from build123d import *

# Parameters (mm, degrees)
SKETCH1_W           = 60.96
SKETCH1_H           = 60.96
SKETCH1_R           = 1
SKETCH1_R_2         = 0.5
BOSS_EXTRUDE1_DEPTH = 1.5
SKETCH1_3_R         = 0.5
CUT_EXTRUDE1_DEPTH  = 0.75


with BuildPart() as part:
    # Sketch1 → Boss-Extrude1 (new body)
    with BuildSketch(Plane(origin=(0, 0, 0), x_dir=(1, 0, 0), z_dir=(0, 1, 0))):
        with Locations((30.48, 30.48)):
            Rectangle(SKETCH1_W, SKETCH1_H)
        with Locations(Location((25.4, 40.64, 0), (0, 0, 270))):  # turned: the seam where the file's is
            Circle(SKETCH1_R, mode=Mode.SUBTRACT)
        with Locations(Location((25.4, 25.4, 0), (0, 0, 270))):  # turned: the seam where the file's is
            Circle(SKETCH1_R, mode=Mode.SUBTRACT)
        with Locations((10.16, 58.42)):
            Circle(SKETCH1_R_2, mode=Mode.SUBTRACT)
        with Locations(Location((2.54, 2.54, 0), (0, 0, 270))):  # turned: the seam where the file's is
            Circle(SKETCH1_R, mode=Mode.SUBTRACT)
        with Locations((10.16, 2.54)):
            Circle(SKETCH1_R_2, mode=Mode.SUBTRACT)
        with Locations((58.42, 15.24)):
            Circle(SKETCH1_R_2, mode=Mode.SUBTRACT)
        with Locations((58.42, 45.72)):
            Circle(SKETCH1_R_2, mode=Mode.SUBTRACT)
        with Locations(Location((2.54, 58.42, 0), (0, 0, 270))):  # turned: the seam where the file's is
            Circle(SKETCH1_R, mode=Mode.SUBTRACT)
        with Locations((10.16, 58.42)):
            Circle(SKETCH1_R_2)
        with Locations((58.42, 45.72)):
            Circle(SKETCH1_R_2)
        with Locations((58.42, 15.24)):
            Circle(SKETCH1_R_2)
        with Locations((10.16, 2.54)):
            Circle(SKETCH1_R_2)
    extrude(amount=BOSS_EXTRUDE1_DEPTH)

    # Sketch1_3 → Cut-Extrude1 (cut)
    with BuildSketch(Plane(origin=(0, 0, 0), x_dir=(1, 0, 0), z_dir=(0, 1, 0))):
        with Locations(Location((10.16, 2.54, 0), (0, 0, 270))):  # turned: the seam where the file's is
            Circle(SKETCH1_3_R)
        with Locations(Location((58.42, 15.24, 0), (0, 0, 270))):  # turned: the seam where the file's is
            Circle(SKETCH1_3_R)
        with Locations(Location((58.42, 45.72, 0), (0, 0, 90))):  # turned: the seam where the file's is
            Circle(SKETCH1_3_R)
        with Locations(Location((10.16, 58.42, 0), (0, 0, 90))):  # turned: the seam where the file's is
            Circle(SKETCH1_3_R)
    extrude(amount=CUT_EXTRUDE1_DEPTH, mode=Mode.SUBTRACT)


solid = part.part
The listing builds one solid part. Answer for the finished solid, in the listing's coordinates (mm). Give positions to 0.01 mm unless a question says otherwise; leave off trailing zeros. Write each loop counter-clockwise with the first axis right and the second up, starting at its lowest first coordinate (ties: lowest second). Pieces come first, ordered by that corner, then holes.
1) Section B-B (z = -25.4) is taken. Write down the section's boundary in (x, y).
2) Find the intervals of material crossed by L1, parallel to X at y = 0.7, z = -2.54; L2, parallel to Z at x = 58.42, y = 0.6; L3, parallel to X at y = 0.2, z = -45.72, in increasing order.
3) Section A-A (x = 2.54) is taken. Write down the section's boundary in (y, z), and give its area (3 significant figures).
4) For a pull along X with two mould halves and no side action, classify faces 1 (the face through (0, 1, -30)), 2 (the face through (2.84, 0.74, -57.466)), 3 (the face through (30, 0, -31)) as pulls with the +X half, pulls with the -X half, needs draft (parallel to the pull), parting line crosses it, or undercut.
5) Given P1, Ø1.2, axis at x = 25.4, z = -40.64, coming from the -Y side, flat-ended and moving along its own axis, determine where the tip first touches the part or whether it passes through.
Response:
1. outline: (0, 0) - (24.4, 0) - (24.4, 1.5) - (0, 1.5) - close; (26.4, 0) - (60.96, 0) - (60.96, 1.5) - (26.4, 1.5) - close
2. L1: x = 0 to 1.54, 3.54 to 9.66, 10.66 to 60.96
2. L2: z = -60.96 to -46.22, -45.22 to -15.74, -14.74 to 0
2. L3: x = 0 to 57.92, 58.92 to 60.96
3. outline: (0, -60.96) - (1.5, -60.96) - (1.5, -59.42) - (0, -59.42) - close; (0, -57.42) - (1.5, -57.42) - (1.5, -3.54) - (0, -3.54) - close; (0, -1.54) - (1.5, -1.54) - (1.5, 0) - (0, 0) - close
3. area: 85.4 mm2
4. face 1: pulls with the -X half
4. face 2: undercut
4. face 3: needs draft
5. P1: passes through
